from build123d import *

# Parameters (mm, degrees)
SKETCH1_R           = 2.032
BOSS_EXTRUDE1_DEPTH = 17.526
SKETCH2_W           = 9.398
SKETCH2_H           = 2.159
BOSS_EXTRUDE2_DEPTH = 7.62
CHAMFER1_SIZE       = 6.35
SKETCH3_R           = 1.524
BOSS_EXTRUDE3_DEPTH = 11
FILLET1_R           = 0.508


with BuildPart() as part:
    # Sketch1 → Boss-Extrude1 (new body)
    with BuildSketch(Plane(origin=(0, 0, 0), x_dir=(1, 0, 0), z_dir=(0, 1, 0))):
        with Locations(Location((0, 0, 0), (0, 0, 270))):
            Circle(SKETCH1_R)
    extrude(amount=BOSS_EXTRUDE1_DEPTH)

    # Sketch2 → Boss-Extrude2 (add)
    with BuildSketch(Plane.XZ):
        with Locations((4.699, 0)):
            Rectangle(SKETCH2_W, SKETCH2_H)
    extrude(amount=-BOSS_EXTRUDE2_DEPTH)

    # Chamfer1
    chamfer1_edges = [part.edges().sort_by_distance(p)[0] for p in [
        (9.398, 7.62, 0),
    ]]
    chamfer(chamfer1_edges, length=CHAMFER1_SIZE)

    # Sketch3 → Boss-Extrude3 (add)
    with BuildSketch(Plane(origin=(0, 17.526, 0), x_dir=(1, 0, 0), z_dir=(0, 1, 0))):
        with Locations(Location((0, 0, 0), (0, 0, 270))):
            Circle(SKETCH3_R)
    extrude(amount=BOSS_EXTRUDE3_DEPTH)

    # Fillet1
    fillet1_edges = [part.edges().sort_by_distance(p)[0] for p in [
        (0, 28.526, -1.524),
    ]]
    fillet(fillet1_edges, radius=FILLET1_R)


solid = part.part
CAD build for the part. Positions are in the model's coordinates, mm. A direction names the side the tool comes from. Round coordinates to 2 decimals unless told otherwise and drop trailing zeros. Write each loop counter-clockwise with the first axis right and the second up, starting at its lowest first coordinate (ties: lowest second). Pieces come first, ordered by that corner, then holes.
(1) Slice it at C-C, the plane y = 20.75. Write the cut outline in (x, z), and give its area (3 significant figures).
(2) Slice it at B-B, the plane x = 0. Write the cut outline in (y, z).
(3) 3-axis set-ups, long thin cutter, end or side, ignore diameter. For faces 1 (the face through (1.285, 22.699, 0.819)), 2 (the face through (6.18, 4.49, -0.02)), 3 (the face through (5, 3, 1.08)), 4 (the face through (5, 3, -1.08)), 5 (the face through (4, 0, 0)): which of +Z, -Z, +X, -X, +Y, -Y reach the whole face in a straight line?
(4) Drop flat-ended pins along their axis: P1, Ø2, axis at x = 8, z = 0.5, coming from the +Y side; P2, Ø2, axis at y = 13, z = -0.5, coming from the +X side; P3, Ø6, axis at x = 6, y = 7, coming from the -Z side. Give the stop position or say it passes through.
(5) Probe line 1 along Y through (x, z) = (2.5, -0.1); line 2 along Y through (x, z) = (0.5, 1.8); line 3 along X through (y, z) = (2.75, -1.4). List the from-to ranges inside material, lowest first.
(6) Slice it at D-D, the plane x = 2.75. Write the cut outline in (y, z).
(7) Slice it at A-A, the plane z = 0. Write the cut outline in (x, y), and give its area (3 significant figures).
From the geometry:
1. outline: circle Ø3.05 at (0, 0)
1. area: 7.30 mm2
2. outline: (0, -2.03) - (17.53, -2.03) - (17.53, -1.52) - (28.02, -1.52) arc R0.51 ccw to (28.53, -1.02) - (28.53, 1.02) arc R0.51 ccw to (28.02, 1.52) - (17.53, 1.52) - (17.53, 2.03) - (0, 2.03) - close
3. face 1: +Y
3. face 2: +Z, -Z, +X, +Y
3. face 3: +Z, +X, +Y, -Y
3. face 4: -Z, +X, +Y, -Y
3. face 5: +Z, -Z, +X, -X, -Y
4. P1: stops at y = 3.67
4. P2: stops at x = 2.03
4. P3: stops at z = -1.08
5. line 1: y = 0 to 7.62
5. line 2: y = 0 to 17.53
5. line 3: x = -1.47 to 1.47
6. outline: (0, -1.08) - (7.62, -1.08) - (7.62, 1.08) - (0, 1.08) - close
7. outline: (-2.03, 0) - (9.4, 0) - (9.4, 1.27) - (3.05, 7.62) - (2.03, 7.62) - (2.03, 17.53) - (1.52, 17.53) - (1.52, 28.02) arc R0.51 ccw to (1.02, 28.53) - (-1.02, 28.53) arc R0.51 ccw to (-1.52, 28.02) - (-1.52, 17.53) - (-2.03, 17.53) - close
7. area: 141 mm2
